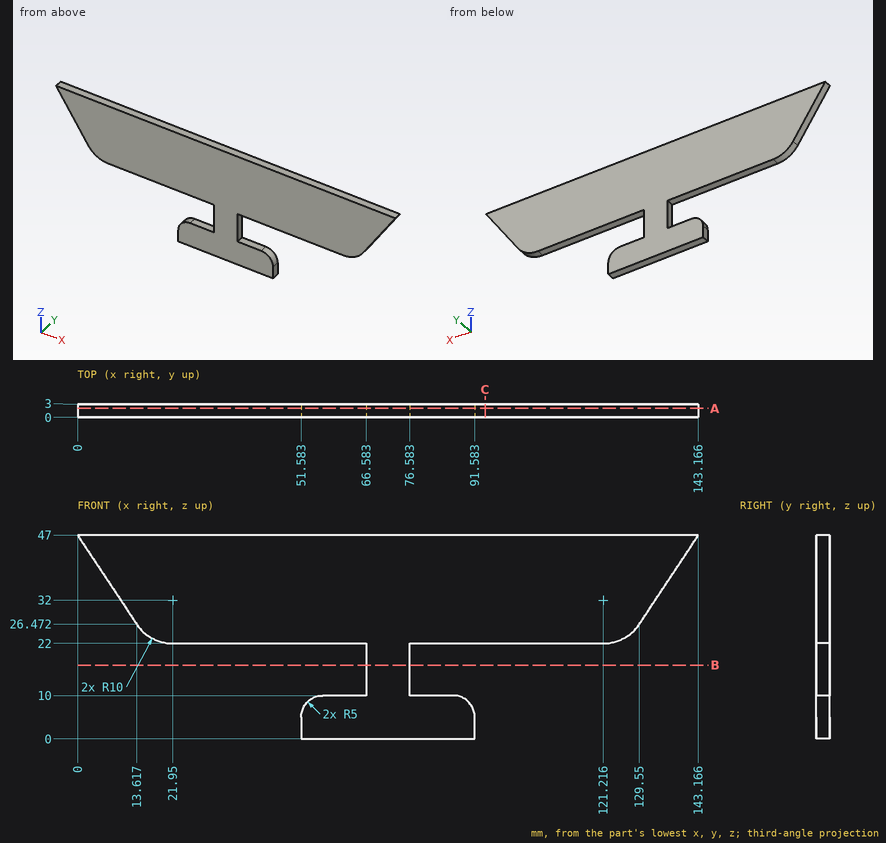
Geometry: see drawing. Coordinates: mm, zero at the bounding-box minimum. Round coordinates to 2 decimals unless told otherwise and drop trailing zeros. Write each loop counter-clockwise with the first axis right and the second up, starting at its lowest first coordinate (ties: lowest second). Pieces come first, ordered by that corner, then holes.
Item 1: Section query A-A (y = 2). Return loops of the section in (x, z), plus the area to 4 significant figures.
Item 2: Pin query (flat end, axial travel): P1, Ø1.5, axis at y = 1, z = 19, coming from the +X side; P2, Ø1.5, axis at y = 2, z = 2.5, coming from the +X side; P3, Ø1.5, axis at x = 45.5, y = 1.5, coming from the -Z side. Return the tip coordinate at first contact, or that it passes through.
Item 3: Material intervals for L1, parallel to Z at x = 47, y = 1.7; L2, parallel to X at y = 0.8, z = 10.5; L3, parallel to X at y = 1.2, z = 3, sorted ascending.
Item 4: Section query C-C (x = 94). Return loops of the section in (y, z).
Item 5: Section query B-B (z = 17). Return loops of the section in (x, y).
Completed:
1. outline: (0, 47) - (13.62, 26.47) arc R10 ccw to (21.95, 22) - (66.58, 22) - (66.58, 10) - (56.58, 10) arc R5 ccw to (51.58, 5) - (51.58, 0) - (91.58, 0) - (91.58, 5) arc R5 ccw to (86.58, 10) - (76.58, 10) - (76.58, 22) - (121.22, 22) arc R10 ccw to (129.55, 26.47) - (143.17, 47) - close
1. area: 3,665 mm2
2. P1: stops at x = 76.58
2. P2: stops at x = 91.58
2. P3: stops at z = 22
3. L1: z = 22 to 47
3. L2: x = 66.58 to 76.58
3. L3: x = 51.58 to 91.58
4. outline: (0, 22) - (3, 22) - (3, 47) - (0, 47) - close
5. outline: (66.58, 0) - (76.58, 0) - (76.58, 3) - (66.58, 3) - close
